```python
from build123d import *

# Parameters (mm, degrees)
F1_DEPTH      = 8
F1_DEPTH_BACK = 15
F2_W          = 3
F2_H          = 2


with BuildPart() as f1:
    # F0 (on Front) → F1 (new body, two sides)
    with BuildSketch(Plane.XZ) as f1_sk:
        with BuildLine():
            Line((-2.350766, 5.86384), (-7, 0))
            Line((-7, 0), (7, 0))
            Line((7, 0), (2.350766, 5.86384))
            ThreePointArc((2.350766, 5.86384), (0, 7), (-2.350766, 5.86384))
        make_face()
    extrude(amount=F1_DEPTH)
    extrude(f1_sk.sketch, amount=-F1_DEPTH_BACK)

    # F2 (on Front) → F3 (revolve, cut)
    with BuildSketch(Plane.XZ):
        Polygon((-3, 6), (-3.5, 2), (-3.5, 0), (0, 0), (0, 6), align=None)
        with Locations((-1.5, 7)):
            Rectangle(F2_W, F2_H)
    revolve(axis=Axis((0, 0, 4.448359), (0, 0, -1)), mode=Mode.SUBTRACT)


solid = f1.part
```
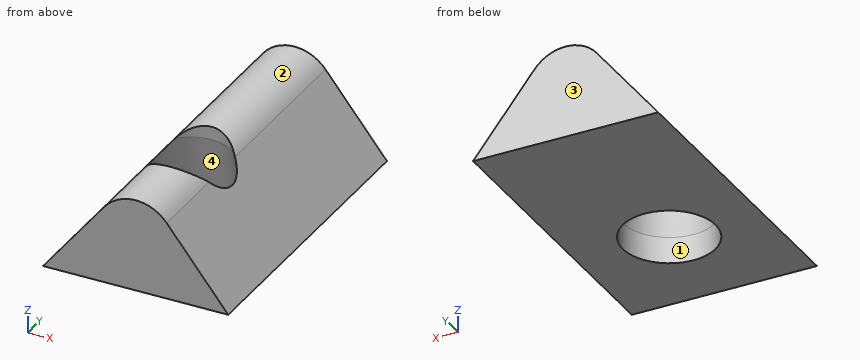
The model under review builds one solid part; all positions refer to its coordinate system, in mm. Face numbers are marked on the shaded views. Round coordinates to 2 decimals unless told otherwise and drop trailing zeros. Write each loop counter-clockwise with the first axis right and the second up, starting at its lowest first coordinate (ties: lowest second). Pieces come first, ordered by that corner, then holes.
(1) We need section A-A on x = 0. Give the boundary of the cut face in (y, z).
(2) Mouldability with a two-part tool opening along X and no side actions: class the marked faces 1, 2, 3 and 4 as +X half, -X half, draft (parallel to the pull), parting line (faces both ways), or undercut.
(3) Insertion check: pin 1 (2 mm diameter, centred on y = 5, z = 5.5, fed in from -X); pin 2 (6 mm diameter, centred on x = -0.5, y = -2.5, fed in from +Z). Each pin has a flat end and moves straight along its axis. Give the tip position at first contact, or say it passes through.
(4) We need section D-D on x = 4.5. Give the boundary of the cut face in (y, z), and give its area (3 significant figures).
(5) We need section C-C on y = -6.5. Give the boundary of the cut face in (x, z), and give its area (3 significant figures).
(6) We need section B-B on y = 0. Give the boundary of the cut face in (x, z).
(7) Wall thickness on L1, parallel to Y at x = 0, z = 0.85; L2, parallel to Y at x = 1.75, z = 2.25; L3, parallel to X at y = 3, z = 3.25: over which ranges is each line inside the solid? List them lowest first.
Findings below:
1. outline: (-8, 0) - (-3.5, 0) - (-3.5, 2) - (-3, 6) - (-3, 7) - (-8, 7) - close; (3, 6) - (3.5, 2) - (3.5, 0) - (15, 0) - (15, 7) - (3, 7) - close
2. face 1: undercut
2. face 2: parting line
2. face 3: draft
2. face 4: undercut
3. pin 1: stops at x = -3.43
3. pin 2: stops at z = 7
4. outline: (-8, 0) - (15, 0) - (15, 3.15) - (-8, 3.15) - close
4. area: 72.5 mm2
5. outline: (-7, 0) - (7, 0) - (2.35, 5.86) arc R3 ccw to (-2.35, 5.86) - close
5. area: 58.6 mm2
6. outline: (-7, 0) - (-3.5, 0) - (-3.5, 2) - (-3.14, 4.87) - close; (3.14, 4.87) - (3.5, 2) - (3.5, 0) - (7, 0) - close
7. L1: y = -8 to -3.5, 3.5 to 15
7. L2: y = -8 to -2.99, 2.99 to 15
7. L3: x = -4.42 to -1.48, 1.48 to 4.42
